```python
from build123d import *

# Parameters (mm, degrees)
SKETCH1_W           = 28
SKETCH1_H           = 26.15
BOSS_EXTRUDE1_DEPTH = 2
SKETCH12_W          = 52.3
SKETCH12_H          = 9
BOSS_EXTRUDE2_DEPTH = 2
SKETCH13_W          = 30
SKETCH13_H          = 36.1
CUT_EXTRUDE3_DEPTH  = 2
SKETCH15_W          = 2
SKETCH15_H          = 36.1
BOSS_EXTRUDE3_DEPTH = 2


with BuildPart() as part:
    # Sketch1 → Boss-Extrude1 (new body)
    # profile 1 of 2: a face of its own
    with BuildSketch(Plane(origin=(0, 0, 0), x_dir=(1, 0, 0), z_dir=(0, 1, 0))):
        with Locations((14, 39.225)):
            Rectangle(SKETCH1_W, SKETCH1_H)
        with BuildLine():
            Line((19.05, 46.2), (4.05, 46.2))
            ThreePointArc((4.05, 46.2), (2, 48.25), (4.05, 50.3))
            Line((4.05, 50.3), (19.05, 50.3))
            ThreePointArc((19.05, 50.3), (21.1, 48.25), (19.05, 46.2))
        make_face(mode=Mode.SUBTRACT)
    # profile 2 of 2: a face of its own
    with BuildSketch(Plane(origin=(0, 0, 0), x_dir=(1, 0, 0), z_dir=(0, 1, 0))):
        with Locations((14, 13.075)):
            Rectangle(SKETCH1_W, SKETCH1_H)
        with BuildLine():
            ThreePointArc((4.05, 2), (2, 4.05), (4.05, 6.1))
            Line((4.05, 6.1), (19.05, 6.1))
            ThreePointArc((19.05, 6.1), (21.1, 4.05), (19.05, 2))
            Line((19.05, 2), (4.05, 2))
        make_face(mode=Mode.SUBTRACT)
    extrude(amount=BOSS_EXTRUDE1_DEPTH)

    # Sketch12 → Boss-Extrude2 (add)
    with BuildSketch(Plane(origin=(28, 0, 0), x_dir=(0, 0, -1), z_dir=(1, 0, 0))):
        with Locations((26.15, -2.5)):
            Rectangle(SKETCH12_W, SKETCH12_H)
        with BuildLine():
            Line((6.15, -0.95), (46.15, -0.95))
            ThreePointArc((46.15, -0.95), (48.175, -2.975), (46.15, -5))
            Line((46.15, -5), (6.15, -5))
            ThreePointArc((6.15, -5), (4.125, -2.975), (6.15, -0.95))
        make_face(mode=Mode.SUBTRACT)
    extrude(amount=BOSS_EXTRUDE2_DEPTH)

    # Sketch13 → Cut-Extrude3 (cut)
    with BuildSketch(Plane(origin=(0, 2, 0), x_dir=(1, 0, 0), z_dir=(0, 1, 0))):
        with Locations((15, 26.15)):
            Rectangle(SKETCH13_W, SKETCH13_H)
    extrude(amount=-CUT_EXTRUDE3_DEPTH, mode=Mode.SUBTRACT)

    # Sketch15 → Boss-Extrude3 (add)
    with BuildSketch(Plane(origin=(0, 0, 0), x_dir=(1, 0, 0), z_dir=(0, 1, 0))):
        with Locations((29, 26.15)):
            Rectangle(SKETCH15_W, SKETCH15_H)
    extrude(amount=BOSS_EXTRUDE3_DEPTH)


solid = part.part
```
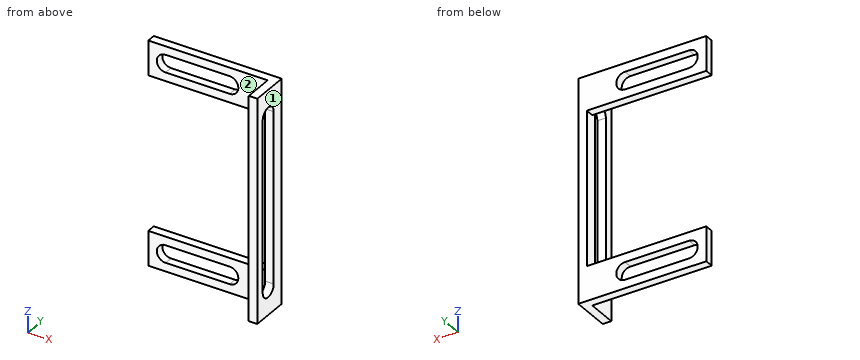
The model under review builds one solid part; all positions refer to its coordinate system, in mm. Face numbers are marked on the shaded views. A direction names the side the tool comes from. Give positions to 0.01 mm unless a question says otherwise; leave off trailing zeros. Write each loop counter-clockwise with the first axis right and the second up, starting at its lowest first coordinate (ties: lowest second). Pieces come first, ordered by that corner, then holes.
(1) To check wall thickness, follow L1, parallel to Z at x = 6, y = 1; L2, parallel to X at y = 1.25, z = -16.5; L3, parallel to Y at x = 1.75, z = -3.5. State the ranges of each line that lie inside material, in increasing order.
(2) Consider section B-B, the plane x = 23.25. Give the boundary of the cut face in (y, z), and give its area (3 significant figures).
(3) Consider section C-C, the plane x = 7. Give the boundary of the cut face in (y, z), and give its area (3 significant figures).
(4) Consider section A-A, the plane z = -36. Give the boundary of the cut face in (x, y), and give its area (3 significant figures).
(5) For P1, Ø1, axis at x = 10, y = 0.5, coming from the +Z side; P2, Ø6.5, axis at x = 16.5, z = -49.5, coming from the -Y side; P3, Ø2, axis at y = -2.5, z = -46, coming from the +X side, all flat-tipped, find the tip position at first contact; note any pin that passes through.
(6) Tool access review of the marked faces 1 and 2: name each direction out of +Z, -Z, +X, -X, +Y, -Y from which nothing blocks a thin tool from reaching the whole face with its end or side.
Returned:
1. L1: z = -52.3 to -50.3, -46.2 to -44.2, -8.1 to -6.1, -2 to 0
1. L2: x = 28 to 30
1. L3: y = 0 to 2
2. outline: (0, -52.3) - (2, -52.3) - (2, -44.2) - (0, -44.2) - close; (0, -8.1) - (2, -8.1) - (2, 0) - (0, 0) - close
2. area: 32.4 mm2
3. outline: (0, -52.3) - (2, -52.3) - (2, -50.3) - (0, -50.3) - close; (0, -46.2) - (2, -46.2) - (2, -44.2) - (0, -44.2) - close; (0, -8.1) - (2, -8.1) - (2, -6.1) - (0, -6.1) - close; (0, -2) - (2, -2) - (2, 0) - (0, 0) - close
3. area: 16.0 mm2
4. outline: (28, -7) - (30, -7) - (30, -5) - (28, -5) - close; (28, -0.95) - (30, -0.95) - (30, 2) - (28, 2) - close
4. area: 9.90 mm2
5. P1: stops at z = 0
5. P2: stops at y = 0
5. P3: passes through
6. face 1: +Z, -Z, +X, +Y, -Y
6. face 2: +Z, -Z, -X, -Y
